from build123d import *

# Parameters (mm, degrees)
F0_W     = 19.05
F0_H     = 19.05
F0_W_2   = 15.875
F0_H_2   = 15.875
F1_DEPTH = 50.8
F3_D     = 5.953125
F3_DEPTH = 6.35
F5_D     = 12.7
F5_DEPTH = 6.35
F7_D     = 5.953125
F7_DEPTH = 6.35


with BuildPart() as f1:
    # F0 (on Front) → F1 (new body)
    with BuildSketch(Plane.XZ):
        Rectangle(F0_W, F0_H)
        Rectangle(F0_W_2, F0_H_2, mode=Mode.SUBTRACT)
    extrude(amount=F1_DEPTH)

    # F3
    with Locations(Plane(origin=(-9.525, 0, 0), x_dir=(0, -1, 0), z_dir=(-1, 0, 0))):
        with Locations((25.4, 0)):
            Hole(F3_D / 2, depth=F3_DEPTH)

    # F5
    with Locations(Plane.YZ.offset(9.525)):
        with Locations((-25.4, 0)):
            Hole(F5_D / 2, depth=F5_DEPTH)

    # F7
    with Locations(Plane.XY.offset(9.525)):
        with Locations((0, -12.7), (0, -38.1)):
            Hole(F7_D / 2, depth=F7_DEPTH)


solid = f1.part
Geometry check sheet. Reference: the model listing, model coordinates, mm. A direction names the side the tool comes from. Coordinates: 2 decimals unless noted, no trailing zeros. Loops run counter-clockwise (first coordinate to the right, second up) from the corner with the lowest first, then second, coordinate; pieces in that order, holes last. Notation, with made-up numbers: (-15, 51.25) - (27, 51.25) arc R23 cw to (27, 66.25) - close; hole circle Ø3 at (74, -37.75). An arc over 180 degrees is marked (long way). Use one line per item in the form item = value. Start each with the question number.
Item 1: Section check A-A, the plane x = 0. Enter the section's corners in (y, z) (1 decimal), and give its area (3 significant figures).
Item 2: Gauge pin test, flat end, axial feed: pin 1 (5 mm diameter, centred on y = -26, z = 2.5, fed in from +X). Record the tip position at first contact, or that the pin passes through.
Item 3: Tool access check on faces 1 (the face through (8.72, -19.056, 0.279)), 2 (the face through (-9.525, -25, 4)), 3 (the face through (-9, -50.8, 0)), 4 (the face through (0.39, -35.15, 8.72)), 5 (the face through (-7.938, -25, 3.4)). Record the directions out of +Z, -Z, +X, -X, +Y, -Y that give a thin tool (end or side, any length) a straight path to the whole face; none if there is none.
Item 4: Section check B-B, the plane y = -34.5. Enter the section's corners in (x, z) (1 decimal), and give its area (3 significant figures).
Item 5: Section check D-D, the plane z = 0. Give the number of separate pieces and of enclosed holes in the cut face, and give its area (3 significant figures).
Item 6: Mould release check, pull along Z, two halves, no side actions. Record for faces 6 (the face through (7.938, -19, -4)), 7 (the face through (9.525, -19, -2)), 8 (the face through (0, -25, 9.525)), 9 (the face through (0, -25, -9.525)): +Z half, -Z half, draft (parallel to the pull), parting line (faces both ways), or undercut.
Item 7: Section check C-C, the plane x = 5.25. Enter the section's corners in (y, z) (1 decimal), and give its area (3 significant figures).
Item 8: Thickness scan on probe 1 along Y at (x, z) = (0, 9); probe 2 along Z at (x, y) = (9.15, -25.4) (3 decimals); probe 3 along X at (y, z) = (-46.5, 5) (1 decimal). Record the ranges inside material, lowest first.
Computed:
q1.outline = (-50.8, -9.5) - (0, -9.5) - (0, -7.9) - (-50.8, -7.9) - close; (-50.8, 7.9) - (-41.1, 7.9) - (-41.1, 9.5) - (-50.8, 9.5) - close; (-35.1, 7.9) - (-15.7, 7.9) - (-15.7, 9.5) - (-35.1, 9.5) - close; (-9.7, 7.9) - (0, 7.9) - (0, 9.5) - (-9.7, 9.5) - close
q1.area = 142 mm2
q2.pin_1 = -7.94
q3.face_1 = +X
q3.face_2 = +Z, -Z, -X, +Y, -Y
q3.face_3 = +Z, -Z, +X, -X, -Y
q3.face_4 = +Z
q3.face_5 = +Y, -Y
q4.outline = (-9.5, -9.5) - (9.5, -9.5) - (9.5, 9.5) - (-9.5, 9.5) - close; hole (-7.9, -7.9) - (7.9, -7.9) - (7.9, 7.9) - (-7.9, 7.9) - close
q4.area = 111 mm2
q5.separate_pieces = 4
q5.enclosed_holes = 0
q5.area = 132 mm2
q6.face_6 = undercut
q6.face_7 = draft
q6.face_8 = +Z half
q6.face_9 = -Z half
q7.outline = (-50.8, -9.5) - (0, -9.5) - (0, -7.9) - (-50.8, -7.9) - close; (-50.8, 7.9) - (0, 7.9) - (0, 9.5) - (-50.8, 9.5) - close
q7.area = 161 mm2
q8.probe_1 = -50.8 to -41.08, -35.12 to -15.68, -9.72 to 0
q8.probe_2 = -9.525 to -6.35, 6.35 to 9.525
q8.probe_3 = -9.5 to -7.9, 7.9 to 9.5
